CAD build for the part. Positions are in the model's coordinates, mm. Face numbers are marked on the shaded views. A direction names the side the tool comes from. Coordinates: 2 decimals unless noted, no trailing zeros. Loops run counter-clockwise (first coordinate to the right, second up) from the corner with the lowest first, then second, coordinate; pieces in that order, holes last. Notation, with made-up numbers: (9.5, 11) - (66.5, 11) arc R22 ccw to (66.5, 38) - close; hole circle Ø9 at (-15, 10). An arc over 180 degrees is marked (long way). Put each result on its own line as item: value.
```python
from build123d import *

# Parameters (mm, degrees)
F2_R      = 2.5
F3_DEPTH  = 3
F4_W      = 3
F4_H      = 35
F4_H_2    = 3
F4_W_2    = 41
F5_DEPTH  = 114
F6_R      = 2.5
F7_DEPTH  = 3
F8_W      = 110
F8_H      = 20
F9_DEPTH  = 3
F10_W     = 47
F10_H     = 26
F10_W_2   = 48
F10_H_2   = 28
F11_DEPTH = 3
F13_DEPTH = 3
F14_SIZE  = 1


with BuildPart() as f3:
    # F2 (on Right) → F3 (new body)
    with BuildSketch(Plane.YZ):
        with BuildLine():
            ThreePointArc((22.5, 35), (21.0355339059, 38.5355339059), (17.5, 40))
            Line((17.5, 40), (-19.5, 40))
            ThreePointArc((-19.5, 40), (-23.0355339059, 38.5355339059), (-24.5, 35))
            Line((-24.5, 35), (-24.5, -38))
            Line((-24.5, -38), (22.5, -38))
            Line((22.5, -38), (22.5, 35))
        make_face()
        with Locations((-12, 34.5)):
            Circle(F2_R, mode=Mode.SUBTRACT)
        with Locations((10, 34.5)):
            Circle(F2_R, mode=Mode.SUBTRACT)
    extrude(amount=F3_DEPTH)

    # F4 (on Right) → F5 (join)
    with BuildSketch(Plane.YZ):
        with Locations((-23, -17.5)):
            Rectangle(F4_W, F4_H)
        with Locations((21, -36.5)):
            Rectangle(F4_W, F4_H_2)
        with Locations((21, -17.5)):
            Rectangle(F4_W, F4_H)
        with Locations((-1, -36.5)):
            Rectangle(F4_W_2, F4_H_2)
        with Locations((-23, -36.5)):
            Rectangle(F4_W, F4_H_2)
    extrude(amount=-F5_DEPTH)

    # F6 (on face) → F7 (join)
    with BuildSketch(Plane(origin=(-114, 0, 0), x_dir=(0, -1, 0), z_dir=(-1, 0, 0))):
        with BuildLine():
            ThreePointArc((24.5, 35), (23.0355339059, 38.5355339059), (19.5, 40))
            Line((19.5, 40), (-17.5, 40))
            ThreePointArc((-17.5, 40), (-21.0355339059, 38.5355339059), (-22.5, 35))
            Line((-22.5, 35), (-22.5, -38))
            Line((-22.5, -38), (24.5, -38))
            Line((24.5, -38), (24.5, 35))
        make_face()
        with Locations((-10, 34.5)):
            Circle(F6_R, mode=Mode.SUBTRACT)
    extrude(amount=F7_DEPTH)

    # F8 (on face) → F9 (join)
    with BuildSketch(Plane.XZ.offset(24.5)):
        with Locations((-57, 10)):
            Rectangle(F8_W, F8_H)
    extrude(amount=-F9_DEPTH)

    # F10 (on face) → F11 (cut, through all)
    with BuildSketch(Plane.XZ.offset(24.5)):
        with Locations((-85.5, -19)):
            Rectangle(F10_W, F10_H)
        with Locations((-28.5, -19)):
            Rectangle(F10_W_2, F10_H_2)
    extrude(amount=-F11_DEPTH, mode=Mode.SUBTRACT)

    # F12 (on face) → F13 (cut, through all)
    with BuildSketch(Plane(origin=(0, 22.5, 0), x_dir=(-1, 0, 0), z_dir=(0, 1, 0))):
        with BuildLine():
            ThreePointArc((82, -26), (82.5857864376, -27.4142135624), (84, -28))
            Line((84, -28), (95, -28))
            ThreePointArc((95, -28), (96.4142135624, -27.4142135624), (97, -26))
            Line((97, -26), (97, -24))
            ThreePointArc((97, -24), (96.4142135624, -22.5857864376), (95, -22))
            Line((95, -22), (84, -22))
            ThreePointArc((84, -22), (82.5857864376, -22.5857864376), (82, -24))
            Line((82, -24), (82, -26))
        make_face()
    extrude(amount=-F13_DEPTH, mode=Mode.SUBTRACT)

    # F14
    f14_edges = [f3.edges().sort_by_distance(p)[0] for p in [
        (-57, -24.5, -38),
        (3, -1, -38),
        (-57, 22.5, -38),
        (-117, -1, -38),
    ]]
    chamfer(f14_edges, length=F14_SIZE)


solid = f3.part
```
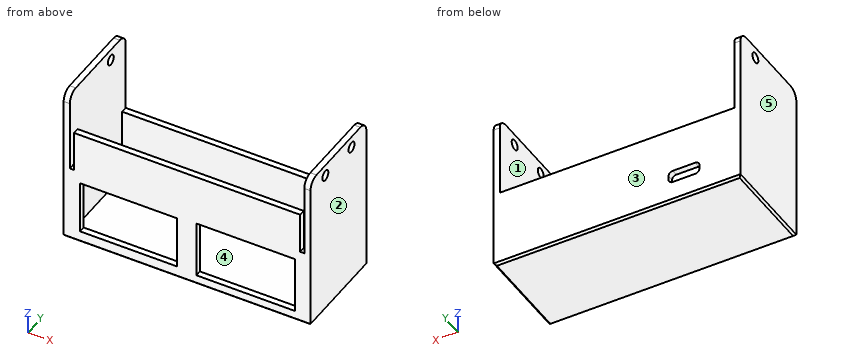
Q1. Tool access for the marked faces 1 and 2: list every direction of +Z, -Z, +X, -X, +Y, -Y with a clear straight run to the whole face (end or side of a thin tool).
Determined:
face 1: +Z
face 2: +Z, -Z, +X, +Y, -Y
Q2. Slice it at C-C, the plane y = 10. Give the cut face in (x, z).
Determined:
outline: (-117, -37) - (-116, -38) - (2, -38) - (3, -37) - (3, 32) - (0, 32) - (0, -35) - (-114, -35) - (-114, 32) - (-117, 32) - close; (-117, 37) - (-114, 37) - (-114, 40) - (-117, 40) - close; (0, 37) - (3, 37) - (3, 40) - (0, 40) - close
Q3. Slice it at B-B, the plane y = -12. Give the cut face in (x, z).
Determined:
outline: (-117, -37) - (-116, -38) - (2, -38) - (3, -37) - (3, 32) - (0, 32) - (0, -35) - (-114, -35) - (-114, 40) - (-117, 40) - close; (0, 37) - (3, 37) - (3, 40) - (0, 40) - close
Q4. Mould opens along Y. For the marked faces 3, 4 and 5 say: +Y half, -Y half, draft (parallel to the pull), parting line (faces both ways), or undercut.
Determined:
face 3: +Y half
face 4: undercut
face 5: draft
Q5. Slice it at D-D, the plane x = -21.5. Give the cut face in (y, z), then the cut area to 3 significant figures.
Determined:
outline: (-24.5, -37) - (-23.5, -38) - (21.5, -38) - (22.5, -37) - (22.5, 0) - (19.5, 0) - (19.5, -35) - (-21.5, -35) - (-21.5, -33) - (-24.5, -33) - close; (-24.5, -5) - (-21.5, -5) - (-21.5, 20) - (-24.5, 20) - close
area: 326 mm2
Q6. Pin check, flat tips, straight feed: pin 1 Ø0.9 at (x, y) = (-88, 21.5) entering from +Z; pin 2 Ø12 at (x, y) = (-81.5, 6) entering from +Z; pin 3 Ø3 at (y, z) = (10, 34.5) entering from +X; pin 4 Ø1.5 at (x, y) = (-34, -23.5) entering from +Z. Stop position of each tip, or through.
Determined:
pin 1: z = 0
pin 2: z = -35
pin 3: through
pin 4: z = 20
Q7. Wall check: L1, parallel to X at y = 5.5, z = 14.5; L2, parallel to Z at x = 1, y = -12; L3, parallel to Z at x = -18, y = 7.5. Give the ranges that are in metal, low to high. Write a range as from..to.
Determined:
L1: -117..-114, 0..3
L2: -38..32, 37..40
L3: -38..-35
Q8. Slice it at A-A, the plane z = 2.5. Give the cut face in (x, y).
Determined:
outline: (-117, -24.5) - (-114, -24.5) - (-114, 22.5) - (-117, 22.5) - close; (-112, -24.5) - (-2, -24.5) - (-2, -21.5) - (-112, -21.5) - close; (0, -24.5) - (3, -24.5) - (3, 22.5) - (0, 22.5) - close
